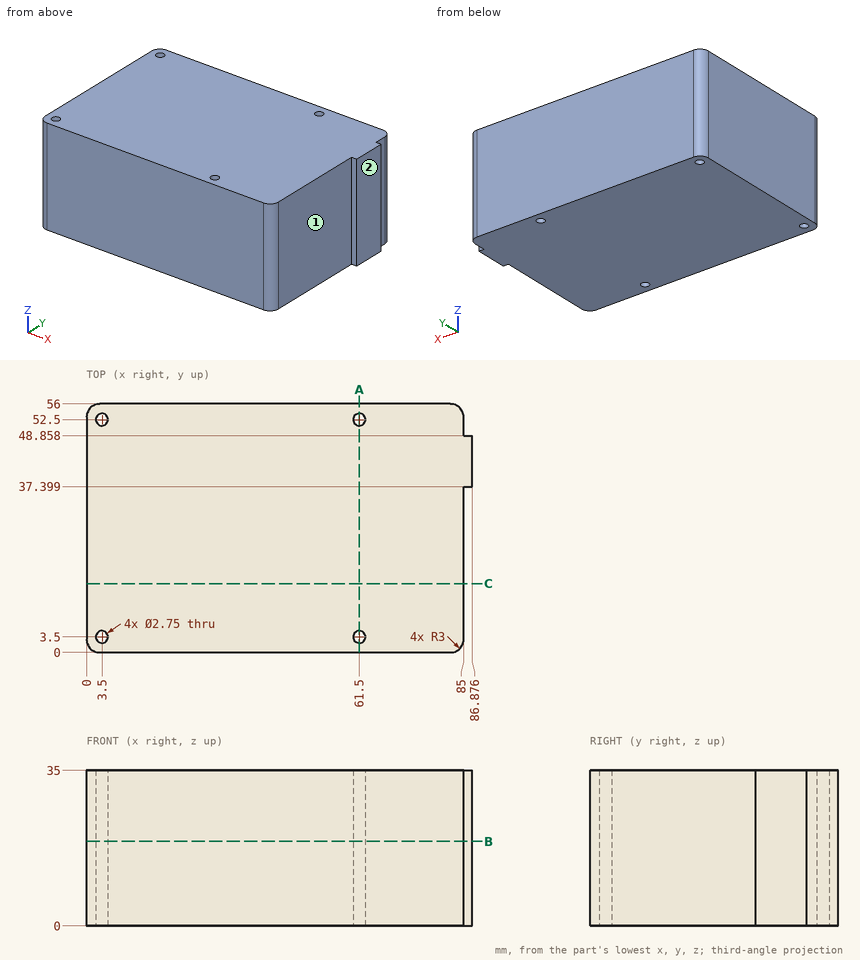
Geometry: see drawing. Coordinates: mm, zero at the bounding-box minimum. A direction names the side the tool comes from. Give positions to 0.01 mm unless a question says otherwise; leave off trailing zeros. Order: outer loops, then holes, each group sorted by start corner. A loop starts at its lowest first (then second) coordinate and runs counter-clockwise, first axis right, second up. Notation, with made-up numbers: (24, -18.75) -> (49, -18.75) arc R7 ccw to (49, -7.75) -> close; hole circle Ø6 at (19, 67.25). An arc over 180 degrees is marked (long way). Write item = value, one per line.
Q1. Set-up query: the marked faces 1 and 2. Return all of +Z, -Z, +X, -X, +Y, -Y with unobstructed straight access to the full face (end or side cutting, diameter ignored); none if empty.
Data:
face_1 = +Z, -Z, +X, -Y
face_2 = +Z, -Z, +X, +Y, -Y
Q2. Cut plane B-B, the plane z = 19. State how many separate pieces and enclosed holes the cut face has, and give its area (3 significant figures).
Data:
separate_pieces = 1
enclosed_holes = 4
area = 4,750 mm^2
Q3. Pin query (flat end, axial travel): pin 1 (1.5 mm diameter, centred on x = 86, z = 23, fed in from +Y); pin 2 (0.9 mm diameter, centred on x = 85.5, z = 9.5, fed in from -Y); pin 3 (10.5 mm diameter, centred on y = 26.5, z = 19.5, fed in from +X). Return the tip coordinate at first contact, or that it passes through.
Data:
pin_1 = 48.86
pin_2 = 37.4
pin_3 = 85
Q4. Cut plane A-A, the plane x = 61.5. Output: boundary loops of the cut face in (y, z) (1 decimal).
Data:
outline = (0, 0) -> (2.1, 0) -> (2.1, 35) -> (0, 35) -> close; (4.9, 0) -> (51.1, 0) -> (51.1, 35) -> (4.9, 35) -> close; (53.9, 0) -> (56, 0) -> (56, 35) -> (53.9, 35) -> close
Q5. Material intervals for line 1 (Y direction, x = 3.5, z = 9) (1 decimal); line 2 (X direction, y = 3, z = 9); line 3 (Y direction, x = 61, z = 12), sorted ascending. Write a range as from..to.
Data:
line_1 = 0..2.1, 4.9..51.1, 53.9..56
line_2 = 0..2.22, 4.78..60.22, 62.78..85
line_3 = 0..2.22, 4.78..51.22, 53.78..56
Q6. Cut plane C-C, the plane y = 15.5. Output: boundary loops of the cut face in (x, z).
Data:
outline = (0, 0) -> (85, 0) -> (85, 35) -> (0, 35) -> close
